Can you work these out from the model? Positions are in its coordinate system, mm. Face numbers are marked on the shaded views. A direction names the side the tool comes from. Give positions to 0.01 mm unless a question says otherwise; leave off trailing zeros. Order: outer loops, then holes, each group sorted by start corner. A loop starts at its lowest first (then second) coordinate and runs counter-clockwise, first axis right, second up. Notation, with made-up numbers: (67.5, 72.25) - (85.5, 72.25) arc R9 ccw to (85.5, 84.25) - close; hole circle Ø10 at (-34.75, 0). An arc over 180 degrees is marked (long way). Answer as CSV lines item,"result".
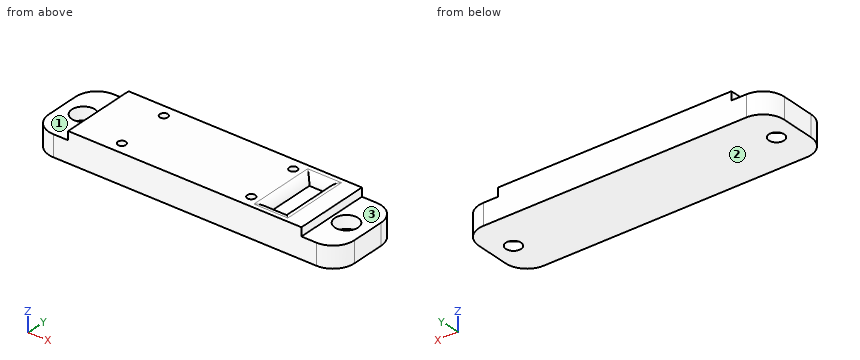
```python
from build123d import *

# Parameters (mm, degrees)
SKETCH_W        = 72
SKETCH_H        = 18
SKETCH_R        = 1.8
PAD_DEPTH       = 7
SKETCH001_R     = 2.75
POCKET_DEPTH    = 5
SKETCH002_W     = 8.5
SKETCH002_H     = 18
SKETCH002_W_2   = 4
SKETCH002_H_2   = 12
POCKET001_DEPTH = 2
SKETCH003_R     = 0.95
POCKET002_DEPTH = 5
FILLET_R        = 5
FILLET001_R     = 1.99


with BuildPart() as part:
    # Sketch → Pad (new body)
    with BuildSketch(Plane.XY):
        Rectangle(SKETCH_W, SKETCH_H)
        with Locations((-31, 0)):
            Circle(SKETCH_R, mode=Mode.SUBTRACT)
        with Locations((31, 0)):
            Circle(SKETCH_R, mode=Mode.SUBTRACT)
    extrude(amount=PAD_DEPTH)

    # Sketch001 (on Face8 of Pad) → Pocket (cut)
    with BuildSketch(Plane.XY.offset(7)):
        with Locations((-31, 0)):
            Circle(SKETCH001_R)
        with Locations((31, 0)):
            Circle(SKETCH001_R)
    extrude(amount=-POCKET_DEPTH, mode=Mode.SUBTRACT)

    # Sketch002 (on Face5 of Pocket) → Pocket001 (cut)
    with BuildSketch(Plane.XY.offset(7)):
        with Locations((-31.75, 0)):
            Rectangle(SKETCH002_W, SKETCH002_H)
        with Locations((31.75, 0)):
            Rectangle(SKETCH002_W, SKETCH002_H)
        with Locations((19.5, 0)):
            Rectangle(SKETCH002_W_2, SKETCH002_H_2)
    extrude(amount=-POCKET001_DEPTH, mode=Mode.SUBTRACT)

    # Sketch003 (on Face11 of Pocket001) → Pocket002 (cut)
    with BuildSketch(Plane.XY.offset(7)):
        with Locations((-17, 6.25)):
            Circle(SKETCH003_R)
        with Locations((-17, -6.25)):
            Circle(SKETCH003_R)
        with Locations((13.5, 6.25)):
            Circle(SKETCH003_R)
        with Locations((13.5, -6.25)):
            Circle(SKETCH003_R)
    extrude(amount=-POCKET002_DEPTH, mode=Mode.SUBTRACT)

    # Fillet
    fillet_edges = [part.edges().sort_by_distance(p)[0] for p in [
        (-36, -9, 2.5),
        (-36, 9, 2.5),
        (36, -9, 2.5),
        (36, 9, 2.5),
    ]]
    fillet(fillet_edges, radius=FILLET_R)

    # Fillet001
    fillet001_edges = [part.edges().sort_by_distance(p)[0] for p in [
        (21.5, 0, 7),
        (19.5, 6, 7),
        (17.5, 0, 7),
        (19.5, -6, 7),
    ]]
    fillet(fillet001_edges, radius=FILLET001_R)


solid = part.part
```
1) I need wall thicknesses on line 1 along Y through (x, z) = (-17, 5.7); line 2 along X through (y, z) = (0, 1.6); line 3 along X through (y, z) = (6.75, 3). Which ranges of each line are inside material? Lowest first, please. Write a range as [from, to].
Answer block:
line 1,"[-9, -7.2], [-5.3, 5.3], [7.2, 9]"
line 2,"[-36, -32.8], [-29.2, 29.2], [32.8, 36]"
line 3,"[-35.18, -17.81], [-16.19, 12.69], [14.31, 35.18]"
2) I want a section at A-A on y = 0. Count the separate pieces of the cut face and the enclosed holes in it, plus the area to 3 significant figures.
Answer block:
separate pieces,"3"
enclosed holes,"0"
area,"413 mm2"
3) I want a section at B-B on x = 13.5. Write out the boundary of the cut face in (y, z).
Answer block:
outline,"(-9, 0) - (9, 0) - (9, 7) - (7.2, 7) - (7.2, 2) - (5.3, 2) - (5.3, 7) - (-5.3, 7) - (-5.3, 2) - (-7.2, 2) - (-7.2, 7) - (-9, 7) - close"
4) I'm going to push flat-ended pins straight in: P1, Ø0.6, axis at x = -16.5, y = -6.5, coming from the +Z side; P2, Ø6, axis at x = -31, y = 0.5, coming from the +Z side. Where does each tip first touch, or does it pass through?
Answer block:
P1,"z = 2"
P2,"z = 5"
5) Which directions (+Z, -Z, +X, -X, +Y, -Y) give clear straight access to the entire face, cutting with the end or side of a thin tool? Please do the marked faces 1, 2 and 3.
Answer block:
face 1,"+Z, -X, +Y, -Y"
face 2,"-Z, +X, -X, +Y, -Y"
face 3,"+Z, +X, +Y, -Y"
